from build123d import *

# Parameters (mm, degrees)
F0_W     = 145
F0_H     = 75
F0_R     = 2.807313
F0_R_2   = 3.341189
F0_R_3   = 3.314808
F0_R_4   = 3.070611
F1_DEPTH = 1.5
F2_W     = 20.444891
F2_H     = 10.22245
F3_DEPTH = 4
F2_W_2   = 3.811762
F2_H_2   = 17.326181
F2_W_3   = 62.547514
F2_H_3   = 6.711255
F4_DEPTH = 8
F2_W_4   = 9.615884
F2_H_4   = 15.152305
F5_DEPTH = 10


with BuildPart() as f1:
    # F0 (on Top) → F1 (new body)
    with BuildSketch(Plane.XY):
        Rectangle(F0_W, F0_H)
        with Locations((-57.613384, -15.869359)):
            Circle(F0_R, mode=Mode.SUBTRACT)
        with Locations((55.052515, -19.9745)):
            Circle(F0_R_2, mode=Mode.SUBTRACT)
        with Locations((-57.561513, 24.321459)):
            Circle(F0_R_3, mode=Mode.SUBTRACT)
        with Locations((43.803934, 26.168576)):
            Circle(F0_R_4, mode=Mode.SUBTRACT)
    extrude(amount=F1_DEPTH)

    # F2 (on face) → F3 (join)
    with BuildSketch(Plane.XY.offset(1.5)):
        with Locations((-35.247806, -30.96582)):
            Rectangle(F2_W, F2_H)
    extrude(amount=F3_DEPTH)

    # F2 (on face) → F4 (join)
    with BuildSketch(Plane.XY.offset(1.5)):
        with Locations((-68.167552, -2.897407)):
            Rectangle(F2_W_2, F2_H_2)
        with Locations((-10.211478, 30.131946)):
            Rectangle(F2_W_3, F2_H_3)
    extrude(amount=F4_DEPTH)

    # F2 (on face) → F5 (join)
    with BuildSketch(Plane.XY.offset(1.5)):
        with Locations((-62.984608, -27.995717)):
            Rectangle(F2_W_4, F2_H_4)
    extrude(amount=F5_DEPTH)


solid = f1.part
Design review of the part built by this model. Coordinates are the model's own, in mm. A direction names the side the tool comes from. Coordinates: 2 decimals unless noted, no trailing zeros. Write each loop counter-clockwise with the first axis right and the second up, starting at its lowest first coordinate (ties: lowest second). Pieces come first, ordered by that corner, then holes. Notation, with made-up numbers: (-33, 23) -> (-26, 23) arc R21 ccw to (-26, 57) -> close; hole circle Ø2 at (-12.5, 19.25). An arc over 180 degrees is marked (long way). Write each question's results on one line, items separated by ' | '. Start each with the question number.
(1) For line 1 along Z through (x, y) = (22.5, 28.5); line 2 along X through (y, z) = (-0.5, 7.5); line 3 along Y through (x, z) = (-10, 3.25), list the stretches that pass through material, from the lowest coordinate up. Write a range as from..to.
(2) Take a section at C-C on x = 44. Write out the cut boundary in (y, z), and give its area (3 significant figures).
(3) Take a section at B-B on y = 31. Write out the cut boundary in (x, z).
(4) Take a section at A-A on z = 3. Write out the cut boundary in (x, y).
(5) The part is to be moulded in two halves that separate along X. For faces 4 (the face through (-60.873, 24.467, 0.74)), 5 (the face through (-11, 30, 9.5)), 6 (the face through (21.062, 30, 5)), say which applies: pulls with the +X half, pulls with the -X half, needs draft (parallel to the pull), parting line crosses it, or undercut.
(6) Clearance check with flat-ended pins moving along their axes: P1, Ø11, axis at x = -38.5, y = -32.5, coming from the +Z side; P2, Ø1.2, axis at y = -33, z = 2.5, coming from the -X side; P3, Ø3.5, axis at x = 43.8, y = 26.17, coming from the -Z side; P4, Ø2, axis at y = -9.5, z = 3.5, coming from the +X side. State where each tip first meets the part, or that it passes through.
(7) Take a section at D-D on x = 19. Write out the cut boundary in (y, z), and give its area (3 significant figures).
(8) Tool access review of faces 1 (the face through (-67.793, -28, 6)), 2 (the face through (-35, -31, 5.5)), 3 (the face through (-11, 33.488, 5)): name each direction out of +Z, -Z, +X, -X, +Y, -Y from which nothing blocks a thin tool from reaching the whole face with its end or side.
Results found:
1) line 1: z = 0..1.5 | line 2: x = -70.07..-66.26 | line 3: y = 26.78..33.49
2) outline: (-37.5, 0) -> (23.1, 0) -> (23.1, 1.5) -> (-37.5, 1.5) -> close; (29.23, 0) -> (37.5, 0) -> (37.5, 1.5) -> (29.23, 1.5) -> close | area: 103 mm2
3) outline: (-72.5, 0) -> (72.5, 0) -> (72.5, 1.5) -> (21.06, 1.5) -> (21.06, 9.5) -> (-41.49, 9.5) -> (-41.49, 1.5) -> (-72.5, 1.5) -> close
4) outline: (-70.07, -11.56) -> (-66.26, -11.56) -> (-66.26, 5.77) -> (-70.07, 5.77) -> close; (-67.79, -35.57) -> (-58.18, -35.57) -> (-58.18, -20.42) -> (-67.79, -20.42) -> close; (-45.47, -36.08) -> (-25.03, -36.08) -> (-25.03, -25.85) -> (-45.47, -25.85) -> close; (-41.49, 26.78) -> (21.06, 26.78) -> (21.06, 33.49) -> (-41.49, 33.49) -> close
5) face 4: undercut | face 5: needs draft | face 6: pulls with the +X half
6) P1: stops at z = 5.5 | P2: stops at x = -67.79 | P3: passes through | P4: stops at x = -66.26
7) outline: (-37.5, 0) -> (37.5, 0) -> (37.5, 1.5) -> (33.49, 1.5) -> (33.49, 9.5) -> (26.78, 9.5) -> (26.78, 1.5) -> (-37.5, 1.5) -> close | area: 166 mm2
8) face 1: +Z, -X, -Y | face 2: +Z, +X, -Y | face 3: +Z, +X, -X, +Y
